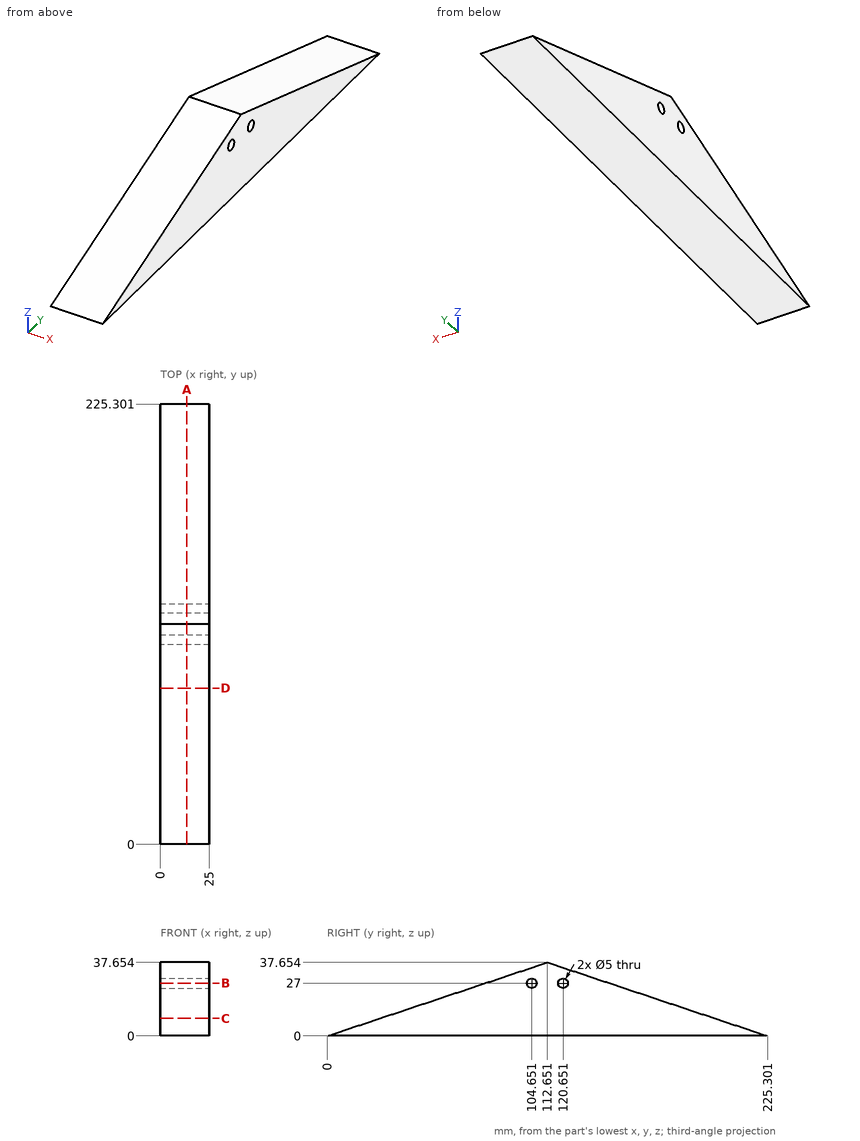
Geometry: see drawing. Coordinates: mm, zero at the bounding-box minimum. Coordinates: 2 decimals unless noted, no trailing zeros. Loops run counter-clockwise (first coordinate to the right, second up) from the corner with the lowest first, then second, coordinate; pieces in that order, holes last. Notation, with made-up numbers: M -16,72 L 8,72 A14 ccw 8,83 Z; hole C 44,-12 d3. An arc over 180 degrees is marked long. Put each result on its own line as item: value. Start each with the question number.
1) Contact query for flat-ended pins moving along their axis: pin 1 Ø4 at (y, z) = (120.65, 27) entering from -X; pin 2 Ø6 at (x, y) = (7, 65) entering from +Z. Output: stop coordinate, or through.
2) Cut plane D-D on y = 80. Return the cut outline in (x, z).
3) Cut plane C-C on z = 9. Return the cut outline in (x, y) (1 decimal).
4) Cut plane A-A on x = 13.5. Return the cut outline in (y, z).
5) Ray query, L1, parallel to Z at x = 8, y = 188; L2, parallel to Z at x = 5.75, y = 69. Return the intervals inside material, ascending. Write a range as from..to.
6) Cut plane B-B on z = 27. Give the number of separate pieces and of enclosed holes in the cut face, then the cut area to 3 significant figures.
The answers:
1. pin 1: passes through
1. pin 2: stops at z = 22.73
2. outline: M 0,0 L 25,0 L 25,26.74 L 0,26.74 Z
3. outline: M 0,26.9 L 25,26.9 L 25,198.4 L 0,198.4 Z
4. outline: M 0,0 L 225.3,0 L 112.65,37.65 Z; hole C 104.65,27 d5; hole C 120.65,27 d5
5. L1: z = 0..12.47
5. L2: z = 0..23.06
6. separate pieces: 3
6. enclosed holes: 0
6. area: 1,340 mm²
